Study the drawing (mm; zero at the part's minimum x, y, z) and answer. Round coordinates to 2 decimals unless told otherwise and drop trailing zeros. Write each loop counter-clockwise with the first axis right and the second up, starting at its lowest first coordinate (ties: lowest second). Pieces come first, ordered by that corner, then holes.
(1) A cutting plane is placed at B-B, the plane z = 38.1. Give the vertices of the cut face in (x, y), and give its area (3 significant figures).
(2) Find the intervals of material crossed by probe 1 along Y at (x, z) = (38.1, 66.25); probe 2 along Z at (x, y) = (14.5, 27.5); probe 3 along Z at (x, y) = (51, 71), in increasing order.
(3) A cutting plane is placed at D-D, the plane y = 39.5. Give the vertices of the cut face in (x, z), and give its area (3 significant figures).
(4) A cutting plane is placed at C-C, the plane x = 56.5. Give the vertices of the cut face in (y, z).
(5) A cutting plane is placed at A-A, the plane x = 38.1. Give the vertices of the cut face in (y, z), and give its area (3 significant figures).
(6) The mould has two halves that part along X. Classify the marked faces 1, 2, 3 and 4: +X half, -X half, draft (parallel to the pull), parting line (faces both ways), or undercut.
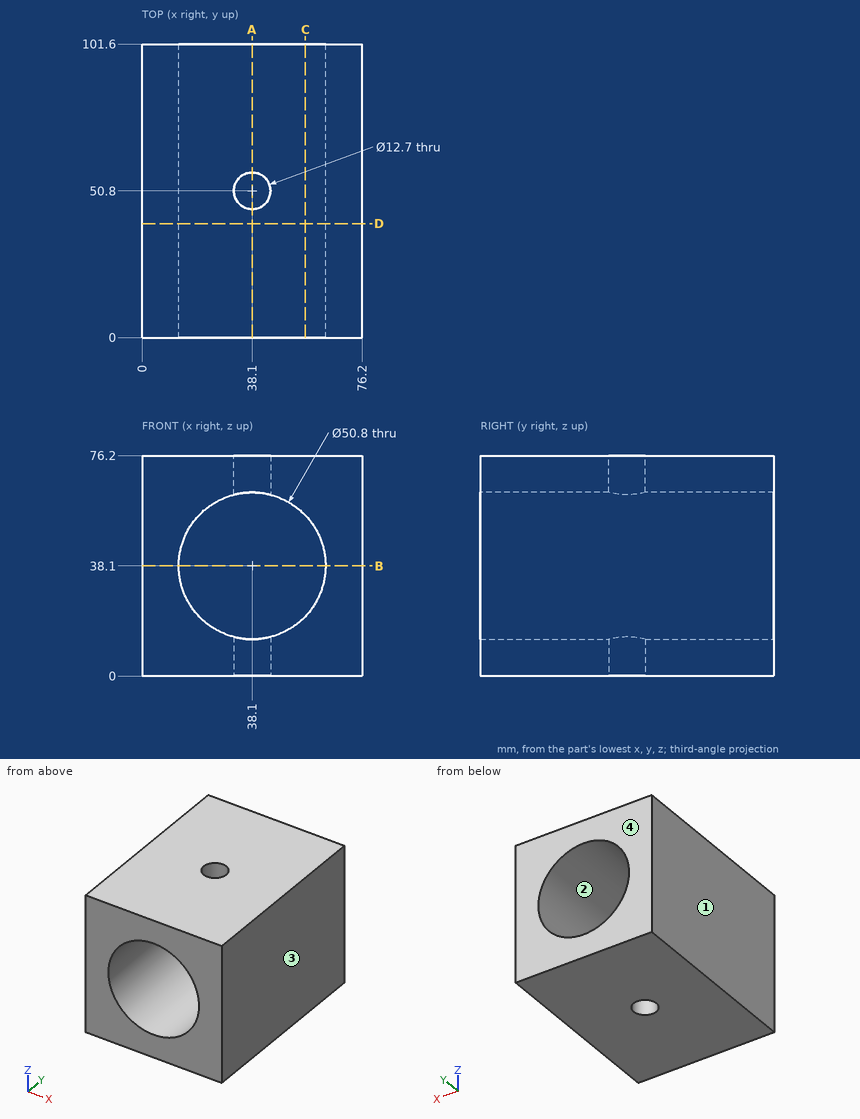
Solutions:
1. outline: (0, 0) - (12.7, 0) - (12.7, 101.6) - (0, 101.6) - close; (63.5, 0) - (76.2, 0) - (76.2, 101.6) - (63.5, 101.6) - close
1. area: 2,580 mm2
2. probe 1: y = 0 to 44.45, 57.15 to 101.6
2. probe 2: z = 0 to 28.71, 47.49 to 76.2
2. probe 3: z = 0 to 16.22, 59.98 to 76.2
3. outline: (0, 0) - (76.2, 0) - (76.2, 76.2) - (0, 76.2) - close; hole circle Ø50.8 at (38.1, 38.1)
3. area: 3,780 mm2
4. outline: (0, 0) - (101.6, 0) - (101.6, 20.59) - (0, 20.59) - close; (0, 55.61) - (101.6, 55.61) - (101.6, 76.2) - (0, 76.2) - close
5. outline: (0, 0) - (44.45, 0) - (44.45, 12.7) - (0, 12.7) - close; (0, 63.5) - (44.45, 63.5) - (44.45, 76.2) - (0, 76.2) - close; (57.15, 0) - (101.6, 0) - (101.6, 12.7) - (57.15, 12.7) - close; (57.15, 63.5) - (101.6, 63.5) - (101.6, 76.2) - (57.15, 76.2) - close
5. area: 2,260 mm2
6. face 1: -X half
6. face 2: undercut
6. face 3: +X half
6. face 4: draft
